```python
from build123d import *

# Parameters (mm, degrees)
SKETCH1_W           = 60
SKETCH1_H           = 60
SKETCH1_R           = 9
SKETCH1_R_2         = 1.5
BOSS_EXTRUDE1_DEPTH = 4
SKETCH4_R           = 3.2
SKETCH4_R_2         = 2.7
BOSS_EXTRUDE6_DEPTH = 34
SKETCH5_W           = 60
SKETCH5_H           = 60
SKETCH5_W_2         = 54
SKETCH5_H_2         = 54
BOSS_EXTRUDE7_DEPTH = 121.7
SKETCH7_W           = 30
SKETCH7_H           = 28
CUT_EXTRUDE1_DEPTH  = 30.7
SKETCH15_R          = 1.5
CUT_EXTRUDE8_DEPTH  = 82
SKETCH17_W          = 54
SKETCH17_H          = 54
CUT_EXTRUDE9_DEPTH  = 38
SKETCH19_R          = 1.5
CUT_EXTRUDE10_DEPTH = 84
SKETCH20_W          = 15
SKETCH20_H          = 15
SKETCH20_R          = 1.5
BOSS_EXTRUDE8_DEPTH = 5


with BuildPart() as part:
    # Sketch1 → Boss-Extrude1 (new body)
    with BuildSketch(Plane.XY):
        with Locations((-9.011180766, -6.125993037)):
            Rectangle(SKETCH1_W, SKETCH1_H)
        with Locations((-9.011180766, -6.125993037)):
            Circle(SKETCH1_R, mode=Mode.SUBTRACT)
        with Locations((-17.995470725, 2.892105033)):
            Circle(SKETCH1_R_2, mode=Mode.SUBTRACT)
        with Locations((-18.051854011, -15.107894967)):
            Circle(SKETCH1_R_2, mode=Mode.SUBTRACT)
        with Locations((0.004529275, 2.892105033)):
            Circle(SKETCH1_R_2, mode=Mode.SUBTRACT)
        with Locations((-0.051854011, -15.107894967)):
            Circle(SKETCH1_R_2, mode=Mode.SUBTRACT)
    extrude(amount=BOSS_EXTRUDE1_DEPTH)

    # Sketch4 → Boss-Extrude6 (add)
    # profile 1 of 3: a face of its own
    with BuildSketch(Plane(origin=(0, 0, 0), x_dir=(-1, 0, 0), z_dir=(0, 0, -1))):
        with Locations(Location((-5.803539584, 2.84752695, 0), (0, 0, 180))):
            Circle(SKETCH4_R)
        with Locations((-5.803539584, 2.84752695)):
            Circle(SKETCH4_R_2, mode=Mode.SUBTRACT)
    # profile 2 of 3: a face of its own
    with BuildSketch(Plane(origin=(0, 0, 0), x_dir=(-1, 0, 0), z_dir=(0, 0, -1))):
        with Locations(Location((24.189837211, 2.217171142, 0), (0, 0, 180))):
            Circle(SKETCH4_R)
        with Locations((24.189837211, 2.217171142)):
            Circle(SKETCH4_R_2, mode=Mode.SUBTRACT)
    # profile 3 of 3: a face of its own
    with BuildSketch(Plane(origin=(0, 0, 0), x_dir=(-1, 0, 0), z_dir=(0, 0, -1))):
        with Locations(Location((8.64724467, -23.442677204, 0), (0, 0, 180))):
            Circle(SKETCH4_R)
        with Locations((8.64724467, -23.442677204)):
            Circle(SKETCH4_R_2, mode=Mode.SUBTRACT)
    extrude(amount=BOSS_EXTRUDE6_DEPTH)

    # Sketch5 → Boss-Extrude7 (add)
    with BuildSketch(Plane.XY.offset(4)):
        with Locations((-9.011180766, -6.125993037)):
            Rectangle(SKETCH5_W, SKETCH5_H)
        with Locations((-9.011180766, -6.125993037)):
            Rectangle(SKETCH5_W_2, SKETCH5_H_2, mode=Mode.SUBTRACT)
    extrude(amount=BOSS_EXTRUDE7_DEPTH)

    # Sketch7 → Cut-Extrude1 (cut)
    with BuildSketch(Plane.XZ.offset(36.125993037)):
        with Locations((-9.011180766, 111.7)):
            Rectangle(SKETCH7_W, SKETCH7_H)
    extrude(amount=-CUT_EXTRUDE1_DEPTH, mode=Mode.SUBTRACT)

    # Sketch15 → Cut-Extrude8 (cut)
    with BuildSketch(Plane.XZ.offset(36.125993037)):
        with Locations(Location((-34.011180766, 115.7, 0), (0, 0, 270))):
            Circle(SKETCH15_R)
        with Locations(Location((15.988819234, 115.7, 0), (0, 0, 270))):
            Circle(SKETCH15_R)
    extrude(amount=-CUT_EXTRUDE8_DEPTH, mode=Mode.SUBTRACT)

    # Sketch17 → Cut-Extrude9 (cut)
    with BuildSketch(Plane.XY.offset(4)):
        with Locations((-9.011180766, -6.125993037)):
            Rectangle(SKETCH17_W, SKETCH17_H)
    extrude(amount=-CUT_EXTRUDE9_DEPTH, mode=Mode.SUBTRACT)

    # Sketch19 → Cut-Extrude10 (cut)
    with BuildSketch(Plane.ZY.offset(39.011180766)):
        with Locations(Location((115.7, 18.874006963, 0), (0, 0, 270))):
            Circle(SKETCH19_R)
        with Locations(Location((115.7, -31.125993037, 0), (0, 0, 270))):
            Circle(SKETCH19_R)
    extrude(amount=-CUT_EXTRUDE10_DEPTH, mode=Mode.SUBTRACT)

    # Sketch20 → Boss-Extrude8 (add)
    # profile 1 of 4: a face of its own
    with BuildSketch(Plane(origin=(0, 0, 0), x_dir=(-1, 0, 0), z_dir=(0, 0, -1))):
        with Locations((-13.488819234, -28.625993037)):
            Rectangle(SKETCH20_W, SKETCH20_H)
        with Locations((-13.488819234, -28.625993037)):
            Circle(SKETCH20_R, mode=Mode.SUBTRACT)
    # profile 2 of 4: a face of its own
    with BuildSketch(Plane(origin=(0, 0, 0), x_dir=(-1, 0, 0), z_dir=(0, 0, -1))):
        with Locations((31.511180766, -28.625993037)):
            Rectangle(SKETCH20_W, SKETCH20_H)
        with Locations((31.511180766, -28.625993037)):
            Circle(SKETCH20_R, mode=Mode.SUBTRACT)
    # profile 3 of 4: a face of its own
    with BuildSketch(Plane(origin=(0, 0, 0), x_dir=(-1, 0, 0), z_dir=(0, 0, -1))):
        with Locations((31.511180766, 16.374006963)):
            Rectangle(SKETCH20_W, SKETCH20_H)
        with Locations((31.511180766, 16.374006963)):
            Circle(SKETCH20_R, mode=Mode.SUBTRACT)
    # profile 4 of 4: a face of its own
    with BuildSketch(Plane(origin=(0, 0, 0), x_dir=(-1, 0, 0), z_dir=(0, 0, -1))):
        with Locations((-13.488819234, 16.374006963)):
            Rectangle(SKETCH20_W, SKETCH20_H)
        with Locations((-13.488819234, 16.374006963)):
            Circle(SKETCH20_R, mode=Mode.SUBTRACT)
    extrude(amount=-BOSS_EXTRUDE8_DEPTH)


solid = part.part
```
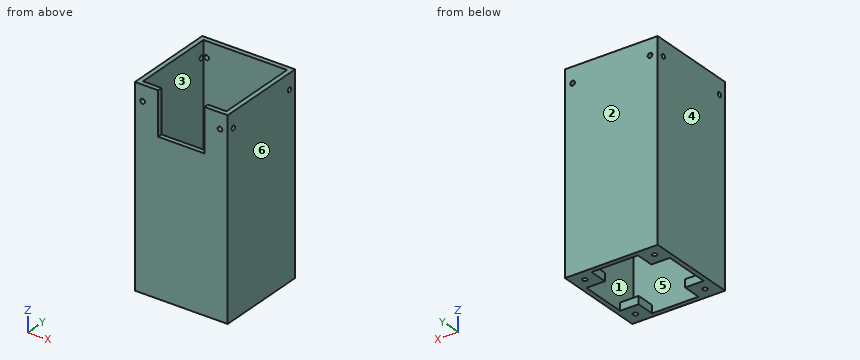
Geometry: final body of the model. Coordinates: model frame, mm. Face numbers are marked on the shaded views. A direction names the side the tool comes from. Give positions to 0.01 mm unless a question says otherwise; leave off trailing zeros. Write each loop counter-clockwise with the first axis right and the second up, starting at its lowest first coordinate (ties: lowest second). Pieces come first, ordered by that corner, then holes.
1. Pin query (flat end, axial travel): P1, Ø5, axis at x = -34.01, z = 115.7, coming from the -Y side; P2, Ø6, axis at x = 9.5, y = -30, coming from the +Z side; P3, Ø1.5, axis at x = -10.5, y = -35, coming from the +Z side. Return the tip coordinate at first contact, or that it passes through.
2. Draft query along X for the marked faces 1, 2, 3 and 4. Return one class per face: released by +X, released by -X, zero draft, split by the parting line, or undercut.
3. Section query C-C, the plane z = 24.5. Return loops of the section in (x, y).
4. Section query B-B, the plane x = 4. Return loops of the section in (y, z), then the cut area to 3 significant figures.
5. Reachability of the marked faces 5 and 6 from +Z, -Z, +X, -X, +Y, -Y: full face, straight path, thin tool, end or side. Return the list, or none.
6. Section query A-A, the plane y = 5.5. Return loops of the section in (x, z).
7. Section query D-D, the plane z = 115.7. Count the separate pieces of the cut face and the enclosed holes in it, then the cut area to 3 significant figures.
8. Line query: probe 1 along X at (y, z) = (23.1, 115.7); probe 2 along X at (y, z) = (-30.5, 18); probe 3 along Y at (x, z) = (17.5, 47.5). Output: solid intervals per line, ascending.
Computed:
1. P1: stops at y = -36.13
1. P2: stops at z = 5
1. P3: stops at z = 97.7
2. face 1: undercut
2. face 2: zero draft
2. face 3: undercut
2. face 4: released by -X
3. outline: (-39.01, -36.13) - (20.99, -36.13) - (20.99, 23.87) - (-39.01, 23.87) - close; hole (-36.01, -33.13) - (17.99, -33.13) - (17.99, 20.87) - (-36.01, 20.87) - close
4. outline: (-36.13, 0) - (-33.13, 0) - (-33.13, 97.7) - (-36.13, 97.7) - close; (20.87, 0) - (23.87, 0) - (23.87, 125.7) - (20.87, 125.7) - close
4. area: 670 mm2
5. face 5: +Z
5. face 6: +Z, -Z, +X, +Y, -Y
6. outline: (-39.01, 0) - (-36.01, 0) - (-36.01, 125.7) - (-39.01, 125.7) - close; (17.99, 0) - (20.99, 0) - (20.99, 125.7) - (17.99, 125.7) - close
7. separate pieces: 9
7. enclosed holes: 0
7. area: 522 mm2
8. probe 1: x = -39.01 to -35.51, -32.51 to 14.49, 17.49 to 20.99
8. probe 2: x = -39.01 to -36.01, 17.99 to 20.99
8. probe 3: y = -36.13 to -33.13, 20.87 to 23.87
